```python
from build123d import *

# Parameters (mm, degrees)
F0_W     = 50
F0_H     = 10
F0_W_2   = 4
F0_H_2   = 4
F0_R     = 1.6
F1_DEPTH = 10
F2_R     = 2.5
F0_W_3   = 56
F0_H_3   = 16
F3_DEPTH = 2
F4_DEPTH = 2
F5_DEPTH = 5
F7_R     = 0.5


# Not quite as in the source:
# - the program builds the solid bodies; features that only make, move or delete a surface that nothing else refers to are left out


with BuildPart() as f1:
    # F0 (on Top) → F1 (new body)
    with BuildSketch(Plane.XY):
        Rectangle(F0_W, F0_H)
        Rectangle(F0_W_2, F0_H_2, mode=Mode.SUBTRACT)
        Rectangle(F0_W_2, F0_H_2)
        Circle(F0_R, mode=Mode.SUBTRACT)
        Circle(F0_R)
    extrude(amount=F1_DEPTH)

    # F2
    f2_edges = [f1.edges().sort_by_distance(p)[0] for p in [
        (-25, -5, 5),
        (-25, 5, 5),
        (25, -5, 5),
        (25, 5, 5),
    ]]
    fillet(f2_edges, radius=F2_R)

    # F0 (on Top) → F3 (join)
    with BuildSketch(Plane.XY):
        Rectangle(F0_W_3, F0_H_3)
        Rectangle(F0_W, F0_H, mode=Mode.SUBTRACT)
    extrude(amount=F3_DEPTH)

    # F0 (on Top) → F4 (join)
    with BuildSketch(Plane.XY):
        Rectangle(F0_W, F0_H)
        Rectangle(F0_W_2, F0_H_2, mode=Mode.SUBTRACT)
    extrude(amount=F4_DEPTH)

    # F0 (on Top) → F5 (join)
    with BuildSketch(Plane.XY):
        Rectangle(F0_W_2, F0_H_2)
        Circle(F0_R, mode=Mode.SUBTRACT)
        Circle(F0_R)
    extrude(amount=-F5_DEPTH)

    # F7
    f7_edges = [f1.edges().sort_by_distance(p)[0] for p in [
        (-2, -2, -2.5),
        (2, -2, -2.5),
        (-2, 2, -2.5),
        (2, 2, -2.5),
    ]]
    fillet(f7_edges, radius=F7_R)


solid = f1.part
```
Can you work these out from the model? Positions are in its coordinate system, mm. A direction names the side the tool comes from. Round coordinates to 2 decimals unless told otherwise and drop trailing zeros. Loops run counter-clockwise (first coordinate to the right, second up) from the corner with the lowest first, then second, coordinate; pieces in that order, holes last.
Item 1: Which directions (+Z, -Z, +X, -X, +Y, -Y) give clear straight access to the entire face, cutting with the end or side of a thin tool? Please do faces 1 (the cylindrical face through (24.287, 4.248, 6.056)), 2 (the flat face through (-25, 0, 6)), 3 (the cylindrical face through (-24.287, 4.248, 6.056)), 4 (the flat face through (0, -2, -2)), 5 (the flat face through (0, 5, 6)).
Item 2: Suppose I cut it at B-B, the plane x = -14. Write out the boundary of the cut face in (y, z).
Item 3: Suppose I cut it at D-D, the plane y = -7. Write out the boundary of the cut face in (x, z), then the cut area to 3 significant figures.
Item 4: Suppose I cut it at A-A, the plane y = -0.5. Write out the boundary of the cut face in (x, z), then the cut area to 3 significant figures.
Item 5: Please list where these lines run through material, in increasing order: L1, parallel to Y at x = 11, z = 4.25; L2, parallel to Z at x = 25.5, y = 1.75; L3, parallel to Z at x = 11, y = -0.5.
Item 6: Suppose I cut it at C-C, the plane z = 2.5. Write out the boundary of the cut face in (x, y), then the cut area to 3 significant figures.
Item 7: Will these pins go through, and if not, where does the flat tip stop? pin 1 Ø1.5 at (y, z) = (0, 7) entering from -X; pin 2 Ø5 at (x, z) = (0.5, 5.5) entering from -Y; pin 3 Ø2.5 at (y, z) = (0.5, -2) entering from -X.
Reported:
1. face 1: +Z, +X, +Y
1. face 2: +Z, -X, +Y, -Y
1. face 3: +Z, -X, +Y
1. face 4: -Z, +X, -X, -Y
1. face 5: +Z, +X, -X, +Y
2. outline: (-8, 0) - (8, 0) - (8, 2) - (5, 2) - (5, 10) - (-5, 10) - (-5, 2) - (-8, 2) - close
3. outline: (-28, 0) - (28, 0) - (28, 2) - (-28, 2) - close
3. area: 112 mm2
4. outline: (-28, 0) - (-2, 0) - (-2, -5) - (2, -5) - (2, 0) - (28, 0) - (28, 2) - (25, 2) - (25, 10) - (-25, 10) - (-25, 2) - (-28, 2) - close
4. area: 532 mm2
5. L1: y = -5 to 5
5. L2: z = 0 to 2
5. L3: z = 0 to 10
6. outline: (-25, -2.5) arc R2.5 ccw to (-22.5, -5) - (22.5, -5) arc R2.5 ccw to (25, -2.5) - (25, 2.5) arc R2.5 ccw to (22.5, 5) - (-22.5, 5) arc R2.5 ccw to (-25, 2.5) - close
6. area: 495 mm2
7. pin 1: stops at x = -25
7. pin 2: stops at y = -5
7. pin 3: stops at x = -2
